For this review, take the finished solid that the model builds, in its own axes (mm). A direction names the side the tool comes from. Coordinates: 2 decimals unless noted, no trailing zeros. Loops run counter-clockwise (first coordinate to the right, second up) from the corner with the lowest first, then second, coordinate; pieces in that order, holes last. Notation, with made-up numbers: M -39,-1 L -26,-1 A31 ccw -26,23 Z; hole C 0.5,18.5 d5. An arc over 180 degrees is marked long. Use one line per item in the form item = value.
Autodesk Fusion 360 part; units mm, degrees
sketch "Sketch1" plane through (0, 0, 0) normal (0, 0, 1) x (1, 0, 0)
  line L0 (-370, 370) -> (370, 370)
  line L1 (370, 370) -> (370, -370)
  line L2 (370, -370) -> (-370, -370)
  line L3 (-370, -370) -> (-370, 370)
  dimension "d1" = 740
  dimension "d2" = 370
  dimension "d3" = 740
  dimension "d4" = 370
extrude "Extrude1" add sketch "Sketch1" along normal blind 20
sketch "Sketch3" plane through (0, 0, 0) normal (0, 0, -1) x (1, 0, 0)
  line L0 (370, 370) -> (-370, 370)
  line L1 (-370, 370) -> (-370, -370)
  line L2 (-370, -370) -> (370, -370)
  line L3 (370, -370) -> (370, 370)
  line L4 (360, 365) -> (340, 365)
  line L5 (340, 365) -> (340, 315)
  line L6 (340, 315) -> (360, 315)
  line L7 (360, 315) -> (360, 365)
  line L8 (360, -315) -> (340, -315)
  line L9 (340, -315) -> (340, -365)
  line L10 (340, -365) -> (360, -365)
  line L11 (360, -365) -> (360, -315)
  line L12 (-340, -315) -> (-360, -315)
  line L13 (-360, -315) -> (-360, -365)
  line L14 (-360, -365) -> (-340, -365)
  line L15 (-340, -365) -> (-340, -315)
  line L16 (-340, 365) -> (-360, 365)
  line L17 (-360, 365) -> (-360, 315)
  line L18 (-360, 315) -> (-340, 315)
  line L19 (-340, 315) -> (-340, 365)
  dimension "d7" = 50
  dimension "d8" = 20
  dimension "d9" = 10
  dimension "d10" = 5
  dimension "d11" = 20
  dimension "d12" = 10
  dimension "d13" = 5
  dimension "d14" = 50
extrude "Extrude2" add sketch "Sketch3" along normal blind 730 contours L4 L5 L6 L7 | L8 L9 L10 L11 | L12 L13 L14 L15 | L16 L17 L18 L19
sketch "Sketch4" plane through (0, 0, 0) normal (0, 0, -1) x (1, 0, 0)
  line L0 (-340, 315) -> (-360, 315)
  line L1 (-360, 315) -> (-360, 365)
  line L2 (-360, 365) -> (-340, 365)
  line L3 (-340, 365) -> (-340, 315)
  line L4 (360, 315) -> (340, 315)
  line L5 (340, 315) -> (340, 365)
  line L6 (340, 365) -> (360, 365)
  line L7 (360, 365) -> (360, 315)
  line L8 (-340, -365) -> (-360, -365)
  line L9 (-360, -365) -> (-360, -315)
  line L10 (-360, -315) -> (-340, -315)
  line L11 (-340, -315) -> (-340, -365)
  line L12 (360, -365) -> (340, -365)
  line L13 (340, -365) -> (340, -315)
  line L14 (340, -315) -> (360, -315)
  line L15 (360, -315) -> (360, -365)
  line L16 (370, 370) -> (-370, 370)
  line L17 (-370, 370) -> (-370, -370)
  line L18 (-370, -370) -> (370, -370)
  line L19 (370, -370) -> (370, 370)
  line L20 (-340, 334) -> (340, 334)
  line L21 (340, 334) -> (340, 319)
  line L22 (340, 319) -> (-340, 319)
  line L23 (-340, 319) -> (-340, 334)
  line L24 (-340, -319) -> (340, -319)
  line L25 (340, -319) -> (340, -334)
  line L26 (340, -334) -> (-340, -334)
  line L27 (-340, -334) -> (-340, -319)
  line L28 (344, 315) -> (359, 315)
  line L29 (359, 315) -> (359, -315)
  line L30 (359, -315) -> (344, -315)
  line L31 (344, -315) -> (344, 315)
  line L32 (-359, 315) -> (-344, 315)
  line L33 (-344, 315) -> (-344, -315)
  line L34 (-344, -315) -> (-359, -315)
  line L35 (-359, -315) -> (-359, 315)
  dimension "d17" = 15
  dimension "d18" = 15
  dimension "d19" = 15
  dimension "d20" = 15
  dimension "d21" = 630
  dimension "d22" = 680
  dimension "d23" = 55
  dimension "d24" = 30
  dimension "d25" = 11
  dimension "d26" = 11
  dimension "d27" = 4
  dimension "d28" = 4
extrude "Extrude3" add sketch "Sketch4" along normal blind 40 contours L0 L10 L32 L33 L34 L35 | L3 L5 L20 L21 L22 L23 | L11 L13 L24 L25 L26 L27 | L4 L14 L28 L29 L30 L31
sketch "Sketch5" plane through (0, 0, 0) normal (0, 0, -1) x (1, 0, 0)
  line L0 (344, -315) -> (344, 315)
  line L1 (344, 315) -> (340, 315)
  line L2 (340, 315) -> (340, 319)
  line L3 (340, 319) -> (-340, 319)
  line L4 (-340, 319) -> (-340, 315)
  line L5 (-340, 315) -> (-344, 315)
  line L6 (-344, 315) -> (-344, -315)
  line L7 (-344, -315) -> (-340, -315)
  line L8 (-340, -315) -> (-340, -319)
  line L9 (-340, -319) -> (340, -319)
  line L10 (340, -319) -> (340, -315)
  line L11 (340, -315) -> (344, -315)
  line L12 (344, -295) -> (320, -319)
  line L13 (344, -280) -> (305, -319)
  line L14 (-320, -319) -> (-344, -295)
  line L15 (-344, -280) -> (-305, -319)
  line L16 (344, 295) -> (320, 319)
  line L17 (344, 280) -> (305, 319)
  line L18 (-320, 319) -> (-344, 295)
  line L19 (-305, 319) -> (-344, 280)
  dimension "d31" = 45
  dimension "d32" = 45
  dimension "d33" = 20
  dimension "d34" = 15
  dimension "d35" = 45
  dimension "d36" = 45
  dimension "d37" = 15
  dimension "d38" = 20
  dimension "d39" = 45
  dimension "d40" = 45
  dimension "d41" = 20
  dimension "d42" = 15
  dimension "d43" = 45
  dimension "d44" = 45
  dimension "d45" = 20
  dimension "d46" = 15
extrude "Extrude4" add sketch "Sketch5" along normal blind 40 contours L0 L9 L12 L13 | L0 L3 L16 L17 | L6 L9 L14 L15 | L3 L6 L18 L19
equation "d2 = ( 740 / 2 ) * 1 mm"
equation "d4 = ( 740 / 2 ) * 1 mm"
equation "d23 = ( ( 740 - 630 ) / 2 ) * 1 mm"
equation "d24 = ( ( 740 - 680 ) / 2 ) * 1 mm"
1. Consider section B-B on y = 219.5. Write out the cut boundary in (x, z).
Computed values:
outline = M -370,0 L -359,0 L -359,-40 L -344,-40 L -344,0 L 344,0 L 344,-40 L 359,-40 L 359,0 L 370,0 L 370,20 L -370,20 Z
2. For pin 1 Ø10 at (x, z) = (351.5, -284) entering from -Y; pin 2 Ø16 at (y, z) = (-305, -25) entering from +X; pin 3 Ø12 at (x, z) = (-12, -26) entering from +Y, all flat-tipped, find the tip position at first contact; note any pin that passes through.
Computed values:
pin_1 = -365
pin_2 = 359
pin_3 = 334
3. Draft analysis for pull direction X (two halves, no side actions). For faces 1 (the face through (360, -340, -360)), 2 (the face through (344, 4, -20)), 3 (the face through (5, 334, -20)), 4 (the face through (-350, -365, -360)), state which applies: +X half, -X half, draft (parallel to the pull), parting line (faces both ways), or undercut.
Computed values:
face_1 = +X half
face_2 = undercut
face_3 = undercut
face_4 = draft
4. Tool access review of faces 5 (the face through (-5, 4, 0)), 6 (the face through (-350, 365, -360)), 7 (the face through (360, 340, -360)), 8 (the face through (350, 340, -730)): name each direction out of +Z, -Z, +X, -X, +Y, -Y from which nothing blocks a thin tool from reaching the whole face with its end or side.
Computed values:
face_5 = -Z
face_6 = -Z, +X, -X, +Y
face_7 = -Z, +X, +Y, -Y
face_8 = -Z, +X, -X, +Y, -Y
5. Wall thickness on line 1 along X through (y, z) = (-326.5, -285); line 2 along Z through (x, y) = (-59.5, -327.5); line 3 along Z through (x, y) = (-231.5, -277): over which ranges is each line inside the solid? List them lowest first. Write a range as from..to.
Computed values:
line_1 = -360..-340, 340..360
line_2 = -40..20
line_3 = 0..20
6. Consider section C-C on x = -269. Write out the cut boundary in (y, z).
Computed values:
outline = M -370,0 L -334,0 L -334,-40 L -319,-40 L -319,0 L 319,0 L 319,-40 L 334,-40 L 334,0 L 370,0 L 370,20 L -370,20 Z
7. Consider section A-A on z = -599. Write out the cut boundary in (x, y).
Computed values:
outline = M -360,-365 L -340,-365 L -340,-315 L -360,-315 Z; M -360,315 L -340,315 L -340,365 L -360,365 Z; M 340,-365 L 360,-365 L 360,-315 L 340,-315 Z; M 340,315 L 360,315 L 360,365 L 340,365 Z
